from build123d import *

# Parameters (mm, degrees)
F1_DEPTH = 250
F3_DEPTH = 250.001
F5_DEPTH = 47.501


with BuildPart() as f1:
    # F0 (on Top) → F1 (new body)
    with BuildSketch(Plane.XY):
        with BuildLine():
            Line((42, 16.186708), (42, 22.186708))
            ThreePointArc((42, 22.186708), (0, 47.5), (-42, 22.186708))
            Line((-42, 22.186708), (-42, 16.186708))
            Line((-42, 16.186708), (42, 16.186708))
        make_face()
    extrude(amount=F1_DEPTH)

    # F2 (on face) → F3 (cut, through all)
    with BuildSketch(Plane.XY.offset(250)):
        with BuildLine():
            ThreePointArc((40, 21.186708), (0, 43.069331), (-40, 21.186708))
            Line((-40, 21.186708), (-40, 16.186708))
            Line((-40, 16.186708), (40, 16.186708))
            Line((40, 16.186708), (40, 21.186708))
        make_face()
    extrude(amount=-F3_DEPTH, mode=Mode.SUBTRACT)

    # F4 (on Front) → F5 (cut, through all)
    with BuildSketch(Plane.XZ):
        Polygon((35, 220), (0, 240), (-35, 220), (0, 200), align=None)
        Polygon((35, 172.5), (0, 192.5), (-35, 172.5), (0, 152.5), align=None)
        Polygon((35, 125), (0, 145), (-35, 125), (0, 105), align=None)
        Polygon((35, 77.5), (0, 97.5), (-35, 77.5), (0, 57.5), align=None)
        Polygon((35, 30), (0, 50), (-35, 30), (0, 10), align=None)
    extrude(amount=-F5_DEPTH, mode=Mode.SUBTRACT)


solid = f1.part
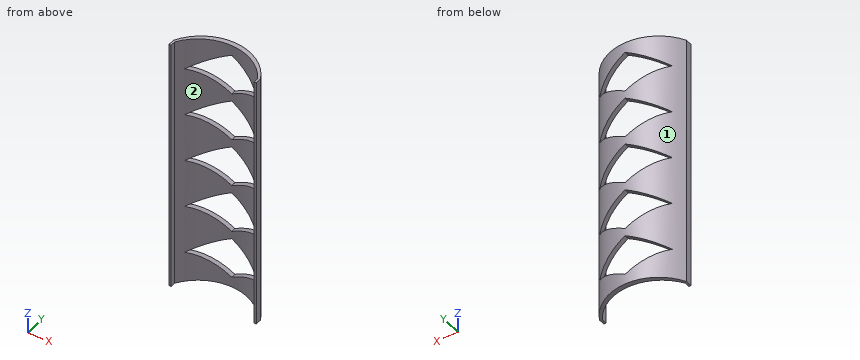
Work out the finished part from the listing and answer in its coordinate system (mm). Face numbers are marked on the shaded views. Round coordinates to 2 decimals unless told otherwise and drop trailing zeros. Loops run counter-clockwise (first coordinate to the right, second up) from the corner with the lowest first, then second, coordinate; pieces in that order, holes last. Notation, with made-up numbers: (-29, -31.75) -> (5, -31.75) arc R30 cw to (5, -1.75) -> close; hole circle Ø1 at (4.25, 10.5). An arc over 180 degrees is marked (long way). Use one line per item in the form item = value.
(1) For a pull along X with two mould halves and no side action, classify the marked faces 1 and 2 as released by +X, released by -X, zero draft, split by the parting line, or undercut.
Answer list:
face_1 = split by the parting line
face_2 = undercut
(2) Find section D-D on z = 140.5. Give the vertices of the cut face in (x, y) (3 decimals), then the cut area to 3 significant figures.
Answer list:
outline = (-42, 16.187) -> (-40, 16.187) -> (-40, 21.187) arc R47.5 cw to (-7.875, 42.412) -> (-7.875, 46.843) arc R47.5 ccw to (-42, 22.187) -> close; (7.875, 42.412) arc R47.5 cw to (40, 21.187) -> (40, 16.187) -> (42, 16.187) -> (42, 22.187) arc R47.5 ccw to (7.875, 46.843) -> close
area = 316 mm2
(3) Find section C-C on x = -21.5. Give the vertices of the cut face in (y, z), then the cut area to 3 significant figures.
Answer list:
outline = (37.92, 0) -> (42.36, 0) -> (42.36, 22.29) -> (37.92, 22.29) -> close; (37.92, 37.71) -> (42.36, 37.71) -> (42.36, 69.79) -> (37.92, 69.79) -> close; (37.92, 85.21) -> (42.36, 85.21) -> (42.36, 117.29) -> (37.92, 117.29) -> close; (37.92, 132.71) -> (42.36, 132.71) -> (42.36, 164.79) -> (37.92, 164.79) -> close; (37.92, 180.21) -> (42.36, 180.21) -> (42.36, 212.29) -> (37.92, 212.29) -> close; (37.92, 227.71) -> (42.36, 227.71) -> (42.36, 250) -> (37.92, 250) -> close
area = 766 mm2
(4) Flat-ended cylindrical pins translate along their axes: P1, Ø2, axis at y = 33, z = 88.5, coming from the +X side; P2, Ø12, axis at y = 28.5, z = 95.5, coming from the -X side; P3, Ø10, axis at x = 32.5, y = 22.5, coming from the -Z side; P4, Ø10, axis at y = 40.5, z = 97, coming from the +X side. Find the tip coordinate at first contact, or state that the pin passes through.
Answer list:
P1 = 35.1
P2 = -41.83
P3 = through
P4 = 31.56
(5) Find section B-B on z = 88. Give the vertices of the cut face in (x, y) (3 decimals), then the cut area to 3 significant figures.
Answer list:
outline = (-42, 16.187) -> (-40, 16.187) -> (-40, 21.187) arc R47.5 cw to (-16.625, 40.065) -> (-16.625, 44.496) arc R47.5 ccw to (-42, 22.187) -> close; (16.625, 40.065) arc R47.5 cw to (40, 21.187) -> (40, 16.187) -> (42, 16.187) -> (42, 22.187) arc R47.5 ccw to (16.625, 44.496) -> close
area = 238 mm2
(6) Straight lines are drawn through the part: line 1 (X direction, y = 20, z = 67.5); line 2 (Z direction, x = -31, y = 35.5); line 3 (X direction, y = 38, z = 46). For each, find the intervals that lie inside material, in ascending order.
Answer list:
line_1 = -42 to -40, 40 to 42
line_2 = 0 to 27.71, 32.29 to 75.21, 79.79 to 122.71, 127.29 to 170.21, 174.79 to 217.71, 222.29 to 250
line_3 = -28.5 to -21.35, 21.35 to 28.5
(7) Find section A-A on y = 19. Give the vertices of the cut face in (x, z).
Answer list:
outline = (-42, 0) -> (-40, 0) -> (-40, 250) -> (-42, 250) -> close; (40, 0) -> (42, 0) -> (42, 250) -> (40, 250) -> close
